```python
from build123d import *

# Parameters (mm, degrees)
F0_R      = 40
F1_DEPTH  = 2
F2_R      = 38.5
F3_DEPTH  = 5
F4_R      = 40
F5_DEPTH  = 50
F7_T      = -2.5
F6_R      = 20
F8_DEPTH  = 10
F9_R      = 2.9
F10_DEPTH = 67.001


with BuildPart() as f1:
    # F0 (on Top) → F1 (new body)
    with BuildSketch(Plane.XY):
        Circle(F0_R)
    extrude(amount=F1_DEPTH)

    # F2 (on face) → F3 (join)
    with BuildSketch(Plane.XY.offset(2)):
        Circle(F2_R)
    extrude(amount=F3_DEPTH)

    # F4 (on face) → F5 (join)
    with BuildSketch(Plane(origin=(0, 0, 0), x_dir=(1, 0, 0), z_dir=(0, 0, -1))):
        Circle(F4_R)
    extrude(amount=F5_DEPTH)

    # F7
    f7_openings = [f1.faces().sort_by_distance(p)[0] for p in [
        (0, 0, 7),
    ]]
    offset(amount=F7_T, openings=f7_openings, kind=Kind.INTERSECTION)

    # F6 (on face) → F8 (join)
    with BuildSketch(Plane(origin=(0, 0, -50), x_dir=(1, 0, 0), z_dir=(0, 0, -1))):
        Circle(F6_R)
    extrude(amount=F8_DEPTH)

    # F9 (on face) → F10 (cut, through all)
    with BuildSketch(Plane(origin=(0, 0, -60), x_dir=(1, 0, 0), z_dir=(0, 0, -1))):
        Circle(F9_R)
    extrude(amount=-F10_DEPTH, mode=Mode.SUBTRACT)


solid = f1.part
```
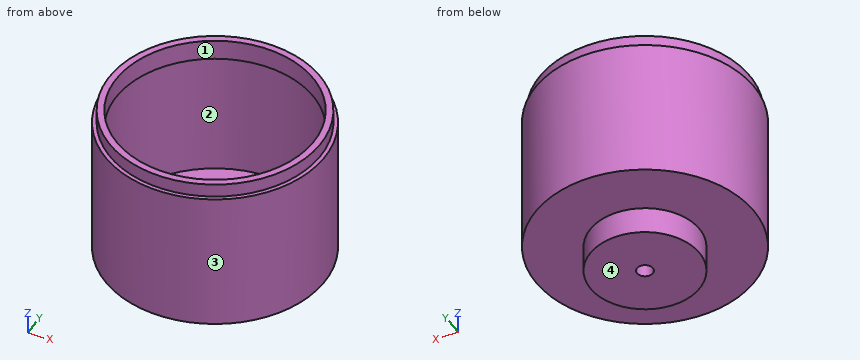
Source: CAD feature listing. Evaluate the final solid. Frame: model axes, mm. Face numbers are marked on the shaded views. Round coordinates to 2 decimals unless told otherwise and drop trailing zeros. Loops run counter-clockwise (first coordinate to the right, second up) from the corner with the lowest first, then second, coordinate; pieces in that order, holes last. Notation, with made-up numbers: M 81,19.25 L 135,19.25 A20 ccw 135,32.25 Z; hole C 68,-38 d5. An arc over 180 degrees is marked long. Use a Markdown table: item, result. Add a question column.
1. Cut plane C-C, the plane z = -52.5. Output: boundary loops of the cut face in (x, y), and give its area (3 significant figures).
2. Pull-direction query (Y, two-part tool) for the marked faces 1, 2, 3 and 4; classes: +Y half, -Y half, draft (parallel to the pull), parting line (faces both ways), or undercut.
3. Ray query, line 1 along X through (y, z) = (0, -54); line 2 along Z through (x, y) = (24, 27); line 3 along Y through (x, z) = (0, -15). Return the intervals inside material, ascending. Write a range as [from, to].
4. Cut plane A-A, the plane x = 0. Output: boundary loops of the cut face in (y, z).
5. Cut plane D-D, the plane y = -17.5. Output: boundary loops of the cut face in (x, z).
6. Contact query for flat-ended pins moving along their axis: pin 1 (7.5 mm diameter, centred on x = 0, y = 0, fed in from +Z); pin 2 (6 mm diameter, centred on x = 8.5, y = 21.5, fed in from -Z); pin 3 (2 mm diameter, centred on x = -8.5, z = -5, fed in from -Y). Output: stop coordinate, or through.
Solution:
| question | item | result |
|---|---|---|
| 1 | outline | C 0,0 d40; hole C 0,0 d5.8 |
| 1 | area | 1,230 mm2 |
| 2 | face 1 | undercut |
| 2 | face 2 | undercut |
| 2 | face 3 | parting line |
| 2 | face 4 | draft |
| 3 | line 1 | x = [-20, -2.9], [2.9, 20] |
| 3 | line 2 | z = [-50, -47.5], [-0.5, 7] |
| 3 | line 3 | y = [-40, -37.5], [37.5, 40] |
| 4 | outline | M -40,-50 L -20,-50 L -20,-60 L -2.9,-60 L -2.9,-47.5 L -37.5,-47.5 L -37.5,-0.5 L -36,-0.5 L -36,7 L -38.5,7 L -38.5,2 L -40,2 Z; M 2.9,-60 L 20,-60 L 20,-50 L 40,-50 L 40,2 L 38.5,2 L 38.5,7 L 36,7 L 36,-0.5 L 37.5,-0.5 L 37.5,-47.5 L 2.9,-47.5 Z |
| 5 | outline | M -35.97,-50 L -9.68,-50 L -9.68,-60 L 9.68,-60 L 9.68,-50 L 35.97,-50 L 35.97,2 L 34.29,2 L 34.29,7 L 31.46,7 L 31.46,-0.5 L 33.17,-0.5 L 33.17,-47.5 L -33.17,-47.5 L -33.17,-0.5 L -31.46,-0.5 L -31.46,7 L -34.29,7 L -34.29,2 L -35.97,2 Z |
| 6 | pin 1 | stops at z = -47.5 |
| 6 | pin 2 | stops at z = -50 |
| 6 | pin 3 | stops at y = -39.29 |
